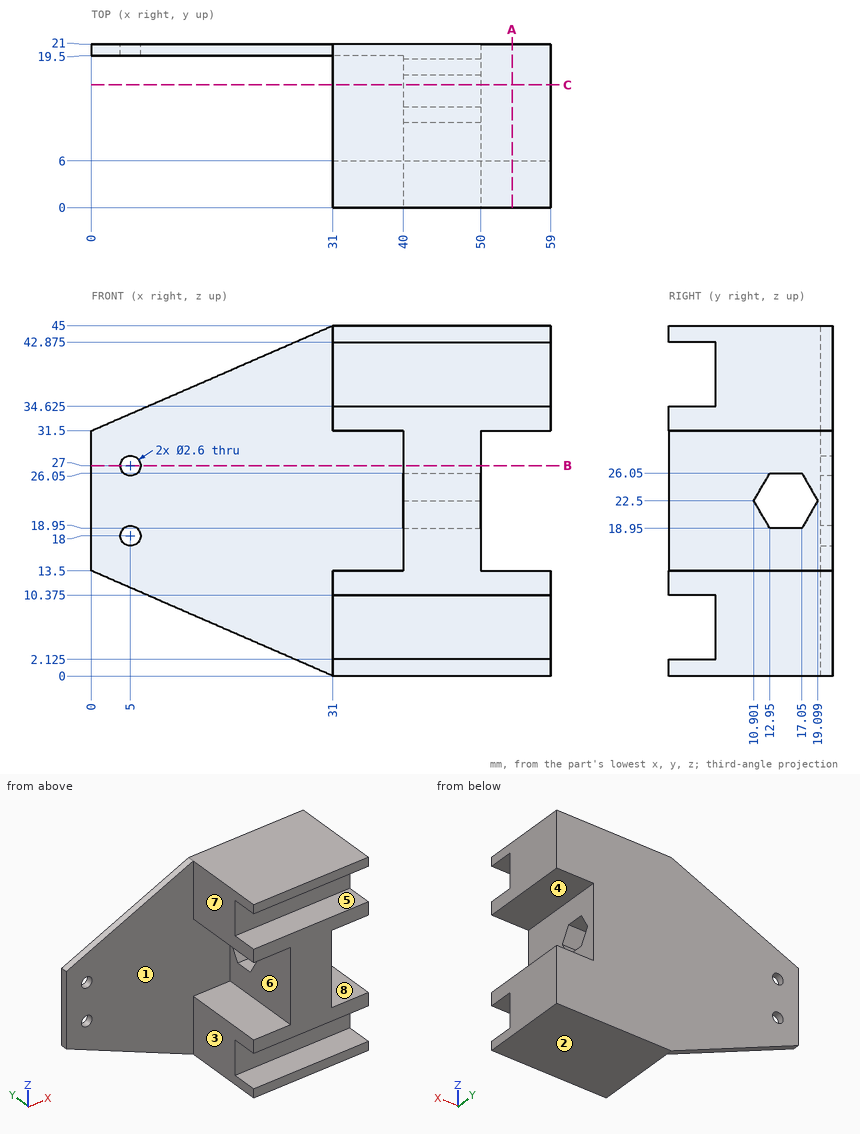
Can you work these out from the drawing? Everything is in mm from the part's minimum corner. A direction names the side the tool comes from. Round coordinates to 2 decimals unless told otherwise and drop trailing zeros. Loops run counter-clockwise (first coordinate to the right, second up) from the corner with the lowest first, then second, coordinate; pieces in that order, holes last. Notation, with made-up numbers: (40.5, 35) -> (87.5, 35) arc R32 ccw to (87.5, 64) -> close; hole circle Ø11 at (58.5, 13). An arc over 180 degrees is marked (long way). One line per question, with ' | ' between items.
(1) If I drill on probe 1 along X at (y, z) = (20.2, 27); probe 2 along Z at (x, y) = (34, 11); probe 3 along Z at (x, y) = (47, 2.5) (1 decimal), over which ranges is the centre line in solid material (lowest first)?
Model answer:
probe 1: x = 0 to 3.7, 6.3 to 50 | probe 2: z = 0 to 13.5, 31.5 to 45 | probe 3: z = 0 to 2.1, 10.4 to 34.6, 42.9 to 45
(2) If we section it at B-B on z = 27: List the corners of the cut face in (x, y) for me.
Model answer:
outline: (0, 19.5) -> (3.7, 19.5) -> (3.7, 21) -> (0, 21) -> close; (6.3, 19.5) -> (40, 19.5) -> (40, 0) -> (50, 0) -> (50, 21) -> (6.3, 21) -> close
(3) For pin 1 Ø8 at (x, z) = (33.5, 29) entering from -Y; pin 2 Ø3 at (y, z) = (9.5, 40) entering from -X; pin 3 Ø12 at (x, y) = (10.5, 10) entering from -Z; pin 4 Ø5.5 at (y, z) = (11.5, 18.5) entering from -X, each with a flat end and sliding along its axis, tell me the tip position at first contact or that it passes through.
Model answer:
pin 1: stops at y = 0 | pin 2: stops at x = 31 | pin 3: passes through | pin 4: stops at x = 40
(4) If we section it at A-A on x = 54: List the corners of the cut face in (y, z) for me (1 decimal), and give its area (3 significant figures).
Model answer:
outline: (0, 0) -> (21, 0) -> (21, 13.5) -> (0, 13.5) -> (0, 10.4) -> (6, 10.4) -> (6, 2.1) -> (0, 2.1) -> close; (0, 31.5) -> (21, 31.5) -> (21, 45) -> (0, 45) -> (0, 42.9) -> (6, 42.9) -> (6, 34.6) -> (0, 34.6) -> close | area: 468 mm^2
(5) For the marked faces 5, 6, 7 and 8, which set-ups out of +Z, -Z, +X, -X, +Y, -Y let a thin tool reach every point of the face, with its end or its side?
Model answer:
face 5: +X, -X, -Y | face 6: -X, -Y | face 7: +Z, -Z, -X, -Y | face 8: +X, +Y, -Y
(6) Thinking about a two-plate mould opening in Z: for the marked faces 1, 2, 3 and 4, which applies, released by +Z, released by -Z, zero draft, split by the parting line, or undercut?
Model answer:
face 1: undercut | face 2: released by -Z | face 3: zero draft | face 4: undercut
(7) If we section it at C-C on y = 15.75: List the corners of the cut face in (x, z) for me, and give its area (3 significant figures).
Model answer:
outline: (31, 0) -> (59, 0) -> (59, 13.5) -> (50, 13.5) -> (50, 18.95) -> (40, 18.95) -> (40, 13.5) -> (31, 13.5) -> close; (31, 31.5) -> (40, 31.5) -> (40, 26.05) -> (50, 26.05) -> (50, 31.5) -> (59, 31.5) -> (59, 45) -> (31, 45) -> close | area: 865 mm^2
